```python
from build123d import *

# Parameters (mm, degrees)
BOSS_EXTRUDE1_DEPTH     = 14.5
CUT_EXTRUDE2_DEPTH      = 36.864327681
CUT_EXTRUDE2_DEPTH_BACK = 36.864327681
SKETCH4_R               = 1.1
SKETCH4_W               = 11
SKETCH4_H               = 11
SKETCH5_R               = 1.25
SKETCH5_R_2             = 1.6
CUT_EXTRUDE3_DEPTH      = 34.797189232
FILLET1_R               = 3


with BuildPart() as part:
    # Sketch1 → Boss-Extrude1 (new, symmetric)
    with BuildSketch(Plane(origin=(0, 0, 0), x_dir=(1, 0, 0), z_dir=(0, 1, 0))):
        Polygon((-7.131727984, 0), (-26, 0), (-26, -4), (-16, -4), (0, -20), (26, -20), (26, 0), (7.131727984, 0), (0, -7.131727984), align=None)
    extrude(amount=BOSS_EXTRUDE1_DEPTH, both=True)

    # Sketch4 → Cut-Extrude2 (cut, two sides: drawn at the far end of the back side and taken through both)
    with BuildSketch(Plane.XY.offset(20).offset(-CUT_EXTRUDE2_DEPTH_BACK)):
        with Locations((21, 10)):
            Circle(SKETCH4_R)
        with Locations((21, -10)):
            Circle(SKETCH4_R)
        with Locations((20.5, 0)):
            Rectangle(SKETCH4_W, SKETCH4_H)
    extrude(amount=CUT_EXTRUDE2_DEPTH + CUT_EXTRUDE2_DEPTH_BACK, mode=Mode.SUBTRACT)

    # Sketch5 → Cut-Extrude3 (cut, through all)
    with BuildSketch(Plane.XY.offset(4)):
        with Locations((-21, 10)):
            Circle(SKETCH5_R)
        with Locations((-21, -10)):
            Circle(SKETCH5_R_2)
    extrude(amount=-CUT_EXTRUDE3_DEPTH, mode=Mode.SUBTRACT)

    # Fillet1
    fillet1_edges = [part.edges().sort_by_distance(p)[0] for p in [
        (-16, 0, 4),
    ]]
    fillet(fillet1_edges, radius=FILLET1_R)


solid = part.part
```
For this review, take the finished solid that the model builds, in its own axes (mm). A direction names the side the tool comes from. Give positions to 0.01 mm unless a question says otherwise; leave off trailing zeros. Write each loop counter-clockwise with the first axis right and the second up, starting at its lowest first coordinate (ties: lowest second). Pieces come first, ordered by that corner, then holes. Notation, with made-up numbers: M -9,55 L 38,55 A5 ccw 38,64 Z; hole C -37.75,-33 d8. An arc over 180 degrees is marked long. One line per item, written item: value.
1) For faces 1 (the cylindrical face through (19.9, 10, 9.9)), 2 (the flat face through (20, 5.5, 10)), 3 (the flat face through (3.616, 0.203, 3.516)), list the 3-axis set-ups (+Z, -Z, +X, -X, +Y, -Y) from which the entire face can be reached by the end or side of a thin tool; tool diameter is ignored.
Results are:
face 1: +Z, -Z
face 2: +Z, -Z, +X
face 3: -Z, +Y, -Y
2) For line 1 (Y direction, x = -21, z = 1.9); line 2 (Y direction, x = 21, z = 8.75); line 3 (Y direction, x = 15.5, z = 13.5), list the stretches that pass through material, from the lowest coordinate up. Write a range as from..to.
Results are:
line 1: y = -14.5..-11.6, -8.4..8.75, 11.25..14.5
line 2: y = -14.5..-11.1, -8.9..-5.5, 5.5..8.9, 11.1..14.5
line 3: y = -14.5..-5.5, 5.5..14.5
3) Take a section at D-D, the plane z = 9. Write out the cut boundary in (x, y), then the cut area to 3 significant figures.
Results are:
outline: M -11,-14.5 L 26,-14.5 L 26,-5.5 L 15,-5.5 L 15,5.5 L 26,5.5 L 26,14.5 L -11,14.5 Z; hole C 21,-10 d2.2; hole C 21,10 d2.2
area: 944 mm²
4) For P1, Ø1.5, axis at x = -3.5, y = -11, coming from the -Z side; P2, Ø2.5, axis at x = -22.5, y = 1.5, coming from the +Z side, all flat-tipped, find the tip position at first contact; note any pin that passes through.
Results are:
P1: stops at z = 2.88
P2: stops at z = 4
5) Take a section at A-A, the plane x = 17. Write out the cut boundary in (y, z).
Results are:
outline: M -14.5,0 L -5.5,0 L -5.5,20 L -14.5,20 Z; M 5.5,0 L 14.5,0 L 14.5,20 L 5.5,20 Z
6) Take a section at B-B, the plane y = 10. Write out the cut boundary in (x, z).
Results are:
outline: M -26,0 L -22.25,0 L -22.25,4 L -26,4 Z; M -19.75,0 L -7.13,0 L 0,7.13 L 7.13,0 L 19.9,0 L 19.9,20 L 0,20 L -15.12,4.88 A3 cw -17.24,4 L -19.75,4 Z; M 22.1,0 L 26,0 L 26,20 L 22.1,20 Z
7) Take a section at C-C, the plane x = -21. Write out the cut boundary in (y, z), then the cut area to 3 significant figures.
Results are:
outline: M -14.5,0 L -11.6,0 L -11.6,4 L -14.5,4 Z; M -8.4,0 L 8.75,0 L 8.75,4 L -8.4,4 Z; M 11.25,0 L 14.5,0 L 14.5,4 L 11.25,4 Z
area: 93.2 mm²
